from build123d import *

# Parameters (mm, degrees)
F1_DEPTH = 68.326
F3_DEPTH = 140.2725
F9_DEPTH = 19.05


with BuildPart() as f1:
    # F0 (on Front) → F1 (new body)
    with BuildSketch(Plane.XZ):
        with BuildLine():
            Line((-308.6435369492, 127.387571028), (-308.6435369492, 73.2729100159))
            Line((-308.6435369492, 73.2729100159), (-168.3720369492, 73.2729100159))
            Line((-168.3720369492, 73.2729100159), (-168.3720369492, 101.8479100159))
            Line((-168.3720369492, 101.8479100159), (-272.5090331009, 150.4077888187))
            ThreePointArc((-272.5090331009, 150.4077888187), (-296.8909470012, 148.8097137516), (-308.6435369492, 127.387571028))
        make_face()
    extrude(amount=F1_DEPTH)

    # F2 (on face) → F3 (cut, through all)
    with BuildSketch(Plane.YZ.offset(-168.3720369492)):
        Polygon((-39.116, 87.6239100159), (-76.0061219335, 87.6239100159), (-76.0061219335, 101.8479100159), (-48.26, 101.8479100159), (-48.26, 161.3023877144), (-91.7473509908, 161.3023877144), (-91.7473509908, 73.2729100159), (-39.116, 73.2729100159), align=None)
    extrude(amount=-F3_DEPTH, mode=Mode.SUBTRACT)

    # F5 (on offset) → F6 (revolve, cut)
    with BuildSketch(Plane(origin=(0, -22.225, 0), x_dir=(-1, 0, 0), z_dir=(0, 1, 0))):
        Polygon((226.816497322, 130.7939626652), (214.7088005788, 126.4077344154), (231.1195903604, 91.2146821577), (239.487580328, 103.6207374686), align=None)
    revolve(axis=Axis((-222.9141954696, -22.225, 108.8112082866), (-0.4226182617, 0, -0.906307787)), mode=Mode.SUBTRACT)

    # F8 (on offset) → F9 (cut)
    with BuildSketch(Plane(origin=(0, -15.748, 0), x_dir=(-1, 0, 0), z_dir=(0, 1, 0))):
        Polygon((320.8571528949, 158.3946817508), (229.5432362601, 158.3946817508), (251.4935369492, 111.3221100159), (320.8571528949, 111.3221100159), align=None)
    extrude(amount=-F9_DEPTH, mode=Mode.SUBTRACT)


solid = f1.part
Can you work these out from the model? Positions are in its coordinate system, mm. A direction names the side the tool comes from. Coordinates: 2 decimals unless noted, no trailing zeros. Loops run counter-clockwise (first coordinate to the right, second up) from the corner with the lowest first, then second, coordinate; pieces in that order, holes last. Notation, with made-up numbers: (82.5, 86) - (119.5, 86) arc R28 ccw to (119.5, 117) - close; hole circle Ø11 at (70.5, -9.5). An arc over 180 degrees is marked (long way). Put each result on its own line as item: value. Start each with the question number.
Item 1: Suppose I cut it at B-B (x = -290.5). Please give me the cut outline in (y, z).
Item 2: Suppose I cut it at D-D (x = -189.5). Please give me the cut outline in (y, z).
Item 3: For pin 1 (14.5 mm diameter, centred on x = -225, y = -49, fed in from -Z); pin 2 (22 mm diameter, centred on x = -236.5, y = -55.5, fed in from +Z); pin 3 (12 mm diameter, centred on x = -261, y = -50.5, fed in from +Z), each with a flat end and sliding along its axis, tell me the tip position at first contact or that it passes through.
Item 4: If I drill on line 1 along Y through (x, z) = (-250, 116); line 2 along Y through (x, z) = (-236, 84.5); line 3 along Y through (x, z) = (-258.5, 107), over which ranges is the centre line in solid material (lowest first)?
Item 5: Suppose I cut it at A-A (z = 137). Please give me the cut outline in (x, y), and give its area (3 significant figures).
Item 6: Which directions (+Z, -Z, +X, -X, +Y, -Y) give clear straight access to the entire face, cutting with the end or side of a thin tool? Please do faces 5 (the face through (-228.537, -22.127, 91.487)), 6 (the face through (-245.806, -25.14, 123.518)), 7 (the face through (-238, -54, 87.624)).
Item 7: If we mould it in two halves opening along Y, with no side actions, what happens to faces 1 (the face through (-255, 0, 105)), 2 (the face through (-274, -34.798, 128)), 3 (the face through (-238, -58, 101.848)), 4 (the face through (-238, -39.116, 80))? For each: +Y half, -Y half, draft (parallel to the pull), parting line (faces both ways), or undercut.
Item 8: Suppose I cut it at C-C (y = -43.5). Please give me the cut outline in (x, z).
Here are the results:
1. outline: (-68.33, 87.62) - (-39.12, 87.62) - (-39.12, 73.27) - (0, 73.27) - (0, 151.73) - (-15.75, 151.73) - (-15.75, 111.32) - (-34.8, 111.32) - (-34.8, 151.73) - (-48.26, 151.73) - (-48.26, 101.85) - (-68.33, 101.85) - close
2. outline: (-68.33, 87.62) - (-39.12, 87.62) - (-39.12, 73.27) - (0, 73.27) - (0, 111.7) - (-48.26, 111.7) - (-48.26, 101.85) - (-68.33, 101.85) - close
3. pin 1: z = 87.62
3. pin 2: z = 137.48
3. pin 3: z = 147.64
4. line 1: -48.26 to -34.8, -15.75 to 0
4. line 2: -39.12 to 0
4. line 3: -48.26 to 0
5. outline: (-306.75, -48.26) - (-243.76, -48.26) - (-243.76, -34.8) - (-306.75, -34.8) - close; (-306.75, -15.75) - (-243.76, -15.75) - (-243.76, 0) - (-306.75, 0) - close
5. area: 1,840 mm²
6. face 5: none
6. face 6: +Z, -X
6. face 7: -Z, +X, -X, -Y
7. face 1: +Y half
7. face 2: undercut
7. face 3: draft
7. face 4: -Y half
8. outline: (-308.64, 87.62) - (-168.37, 87.62) - (-168.37, 101.85) - (-272.51, 150.41) arc R25.4 ccw to (-308.64, 127.39) - close
